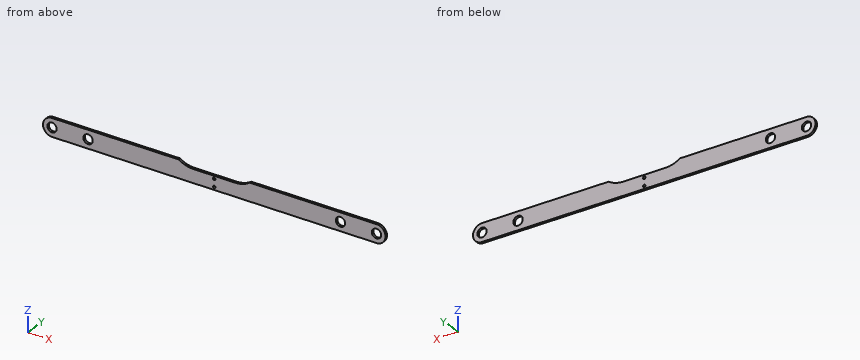
```python
from build123d import *

# Parameters (mm, degrees)
SKETCH5_R           = 3.302
BOSS_EXTRUDE1_DEPTH = 1.5875
SKETCH6_R           = 0.89
CUT_EXTRUDE2_DEPTH  = 121.922062322


with BuildPart() as part:
    # Sketch5 → Boss-Extrude1 (new body)
    with BuildSketch(Plane(origin=(0, 0, 0), x_dir=(1, 0, 0), z_dir=(0, 1, 0))):
        with BuildLine():
            Line((0, 4.75), (-114.3, 4.75))
            ThreePointArc((-114.3, 4.75), (-120.65, -1.6), (-114.3, -7.95))
            Line((-114.3, -7.95), (-25, -7.95))
            ThreePointArc((-25, -7.95), (-20.249761899, -5.569494064), (-15, -4.75))
            Line((-15, -4.75), (0, -4.75))
            Line((0, -4.75), (0, 4.75))
        make_face()
        with Locations(Location((-114.3, -1.6, 0), (0, 0, 270))):
            Circle(SKETCH5_R, mode=Mode.SUBTRACT)
        with Locations(Location((-88.9, -1.6, 0), (0, 0, 270))):
            Circle(SKETCH5_R, mode=Mode.SUBTRACT)
    boss_extrude1 = extrude(amount=BOSS_EXTRUDE1_DEPTH)

    # Mirror1: Boss-Extrude1 across plane
    add(boss_extrude1.mirror(Plane(origin=(0, 1.5875, -4.75), x_dir=(0, 0, 1), z_dir=(-1, 0, 0))))

    # Sketch6 → Cut-Extrude2 (cut, through all)
    with BuildSketch(Plane(origin=(0, 0, 0), x_dir=(1, 0, 0), z_dir=(0, 1, 0))):
        with Locations(Location((0, 2.75, 0), (0, 0, 270))):
            Circle(SKETCH6_R)
        with Locations(Location((0, -2.75, 0), (0, 0, 270))):
            Circle(SKETCH6_R)
    extrude(amount=CUT_EXTRUDE2_DEPTH, mode=Mode.SUBTRACT)


solid = part.part
```
Check sheet for the modelled part. Datum: model origin and axes. Units: mm. Round coordinates to 2 decimals unless told otherwise and drop trailing zeros. Loops run counter-clockwise (first coordinate to the right, second up) from the corner with the lowest first, then second, coordinate; pieces in that order, holes last. Notation, with made-up numbers: M -26.75,-29 L -12.75,-29 A14 cw -12.75,-4 Z; hole C -20,56 d4. An arc over 180 degrees is marked long. Answer as a JSON object with one key per item and string values.
1. Scan lines: line 1 (X direction, y = 0.75, z = 1.6); line 2 (Z direction, x = 0, y = 0.65); line 3 (Z direction, x = 88.9, y = 0.9). Record each from-to range of solid material in increasing order.
Reply:
{"line 1": "x = -120.65 to -117.6, -111 to -92.2, -85.6 to 85.6, 92.2 to 111, 117.6 to 120.65", "line 2": "z = -4.75 to -3.64, -1.86 to 1.86, 3.64 to 4.75", "line 3": "z = -4.75 to -1.7, 4.9 to 7.95"}
2. Section check A-A (x = 88.9). Record the boundary of the cut face in (y, z).
Reply:
{"outline": "M 0,-4.75 L 1.59,-4.75 L 1.59,-1.7 L 0,-1.7 Z; M 0,4.9 L 1.59,4.9 L 1.59,7.95 L 0,7.95 Z"}
3. Gauge pin test, flat end, axial feed: P1, Ø0.8, axis at x = 2.5, y = 0.5, coming from the +Z side. Record the tip position at first contact, or that the pin passes through.
Reply:
{"P1": "stops at z = 4.75"}
4. Section check B-B (y = 0.55). Record the boundary of the cut face in (x, z) (3 decimals).
Reply:
{"outline": "M -114.3,-4.75 L 114.3,-4.75 A6.35 ccw 114.3,7.95 L 25,7.95 A17.225 cw 15,4.75 L -15,4.75 A17.225 cw -25,7.95 L -114.3,7.95 A6.35 ccw Z; hole C -114.3,1.6 d6.604; hole C -88.9,1.6 d6.604; hole C 0,-2.75 d1.78; hole C 0,2.75 d1.78; hole C 88.9,1.6 d6.604; hole C 114.3,1.6 d6.604"}
